Input: part model. Units: mm. Frame: model coordinates. A direction names the side the tool comes from. Coordinates: 2 decimals unless noted, no trailing zeros. Loops run counter-clockwise (first coordinate to the right, second up) from the corner with the lowest first, then second, coordinate; pieces in that order, holes last.
Item 1: Section A-A on z = 20.5. Return loops of the section in (x, y), and give its area (3 significant figures).
Item 2: Reachability of faces 4 (the cylindrical face through (9.573, -0.761, -150.211)), 5 (the flat face through (5, -16, 22)), 6 (the flat face through (5, -16, -112)), 7 (the flat face through (5, -16, -172)), 8 (the flat face through (14, -4, -21)) from +Z, -Z, +X, -X, +Y, -Y: full face, straight path, thin tool, end or side. Return the list, or none.
Item 3: Contact query for flat-ended pins moving along their axis: P1, Ø5, axis at y = -11.5, z = -102.5, coming from the +X side; P2, Ø3.5, axis at y = -18.5, z = -37.5, coming from the -X side; P3, Ø12.5, axis at x = 13, z = -49, coming from the -Y side; P4, Ø2.5, axis at y = -18, z = -54.5, coming from the +X side. Output: stop coordinate, or through.
Item 4: Ray query, line 1 along Y through (x, z) = (2.8, -95.5); line 2 along Y through (x, z) = (10, -54.5); line 3 along Y through (x, z) = (10.75, -92). Return the intervals inside material, ascending.
Item 5: Pull-direction query (Z, two-part tool) for faces 1 (the flat face through (19.289, -5.437, -73.509)), 2 (the cylindrical face through (7.1, -3.25, -56.3)), 3 (the flat face through (14, -4, 21)); classes: released by +Z, released by -Z, zero draft, split by the parting line, or undercut.
Item 6: Section C-C on z = -103. Return loops of the section in (x, y).
Item 7: Section D-D on x = 18.75. Return loops of the section in (y, z), and give its area (3 significant figures).
Item 8: Section B-B on y = -12.75. Return loops of the section in (x, z) (3 decimals).
```python
from build123d import *
from OCP.BRepFilletAPI import BRepFilletAPI_MakeChamfer

# Parameters (mm, degrees)
BOSS_EXTRUDE1_DEPTH     = 10
BOSS_EXTRUDE2_DEPTH     = 12
CUT_EXTRUDE3_DEPTH      = 6
CUT_EXTRUDE3_DEPTH_BACK = 14
SKETCH7_R               = 1.95
SKETCH8_R               = 1.95
CUT_EXTRUDE4_DEPTH      = 4
SKETCH9_R               = 1.5
CUT_EXTRUDE5_DEPTH      = 4
LPATTERN1_COUNT         = 2
LPATTERN1_PITCH         = 75
CHAMFER2_SIZE           = 5.5
CHAMFER2_SIZE2          = 9
CHAMFER3_SIZE           = 7
CHAMFER3_SIZE2          = 2
LPATTERN2_COUNT         = 3
LPATTERN2_PITCH         = 75


with BuildPart() as part:
    # Sketch1 → Boss-Extrude1 (new body)
    with BuildSketch(Plane(origin=(0, 0, 0), x_dir=(1, 0, 0), z_dir=(0, 1, 0))):
        with BuildLine():
            Line((0, -8.075), (0, -31.5))
            Line((0, -31.5), (22, -31.5))
            Line((22, -31.5), (22, 181.5))
            Line((22, 181.5), (0, 181.5))
            Line((0, 181.5), (0, 158.075))
            ThreePointArc((0, 158.075), (8.075, 150), (0, 141.925))
            Line((0, 141.925), (0, 83.075))
            ThreePointArc((0, 83.075), (8.075, 75), (0, 66.925))
            Line((0, 66.925), (0, 8.075))
            ThreePointArc((0, 8.075), (8.075, 0), (0, -8.075))
        make_face()
    extrude(amount=-BOSS_EXTRUDE1_DEPTH)

    # Sketch3 → Boss-Extrude2 (add)
    with BuildSketch(Plane.XZ.offset(10)):
        with BuildLine():
            Line((0, -181.5), (0, -158.075))
            ThreePointArc((0, -158.075), (8.075, -150), (0, -141.925))
            Line((0, -141.925), (0, -83.075))
            ThreePointArc((0, -83.075), (8.075, -75), (0, -66.925))
            Line((0, -66.925), (0, -8.075))
            ThreePointArc((0, -8.075), (8.075, 0), (0, 8.075))
            Line((0, 8.075), (0, 31.5))
            Line((0, 31.5), (5, 31.5))
            Line((5, 31.5), (5, 12.081209583))
            ThreePointArc((5, 12.081209583), (13.075, 0), (5, -12.081209583))
            Line((5, -12.081209583), (5, -62.918790417))
            ThreePointArc((5, -62.918790417), (13.075, -75), (5, -87.081209583))
            Line((5, -87.081209583), (5, -137.918790417))
            ThreePointArc((5, -137.918790417), (13.075, -150), (5, -162.081209583))
            Line((5, -162.081209583), (5, -181.5))
            Line((5, -181.5), (0, -181.5))
        make_face()
    extrude(amount=BOSS_EXTRUDE2_DEPTH)

    # Sketch7 → Cut-Extrude3 (cut, two sides: drawn at the far end of the back side and taken through both)
    with BuildSketch(Plane.ZY.offset(-CUT_EXTRUDE3_DEPTH_BACK)):
        with Locations((-170.5, -4)):
            Circle(SKETCH7_R)
        with Locations((-170.5, -18)):
            Circle(SKETCH7_R)
        with Locations(Location((-129.5, -4, 0), (0, 0, 180))):
            Circle(SKETCH7_R)
        with Locations((-129.5, -18)):
            Circle(SKETCH7_R)
        with Locations((-95.5, -4)):
            Circle(SKETCH7_R)
        with Locations(Location((-54.5, -4, 0), (0, 0, 180))):
            Circle(SKETCH7_R)
        with Locations((-54.5, -18)):
            Circle(SKETCH7_R)
        with Locations((-95.5, -18)):
            Circle(SKETCH7_R)
        with Locations((-20.5, -4)):
            Circle(SKETCH7_R)
        with Locations(Location((20.5, -4, 0), (0, 0, 180))):
            Circle(SKETCH7_R)
        with Locations((20.5, -18)):
            Circle(SKETCH7_R)
        with Locations((-20.5, -18)):
            Circle(SKETCH7_R)
    extrude(amount=CUT_EXTRUDE3_DEPTH + CUT_EXTRUDE3_DEPTH_BACK, mode=Mode.SUBTRACT)

    # Sketch8 → Cut-Extrude4 (cut)
    with BuildSketch(Plane.ZY):
        with Locations((-112.5, -18.5)):
            Circle(SKETCH8_R)
    cut_extrude4 = extrude(amount=-CUT_EXTRUDE4_DEPTH, mode=Mode.SUBTRACT)

    # Sketch9 → Cut-Extrude5 (cut)
    with BuildSketch(Plane.ZY.offset(-4)):
        with Locations((-112.5, -18.5)):
            Circle(SKETCH9_R)
    cut_extrude5 = extrude(amount=-CUT_EXTRUDE5_DEPTH, mode=Mode.SUBTRACT)

    # LPattern1: Cut-Extrude4, Cut-Extrude5 ×2
    with Locations(*[(0, 0, i * LPATTERN1_PITCH) for i in range(1, LPATTERN1_COUNT)]):
        add(cut_extrude4, mode=Mode.SUBTRACT)
        add(cut_extrude5, mode=Mode.SUBTRACT)

    # Chamfer2
    chamfer2_edges = [part.edges().sort_by_distance(p)[0] for p in [
        (22, -10, -75),
    ]]
    chamfer2_side = [part.faces().sort_by_distance(p)[0] for p in [
        (14.183508734, -10, -75),
    ]]
    chamfer(chamfer2_edges, length=CHAMFER2_SIZE, length2=CHAMFER2_SIZE2, reference=chamfer2_side[0])

    # Chamfer3: one chamfer whose edges measure the first distance from different faces: ONE call of the kernel's chamfer builder (chamfer() names one face for all edges)
    chamfer3_edges_1 = [part.edges().sort_by_distance(p)[0] for p in [
        (8.075, -22, 0),
    ]]
    chamfer3_side_1 = [part.faces().sort_by_distance(p)[0] for p in [
        (8.075, -11, 0),
    ]]
    chamfer3_edges_2 = [part.edges().sort_by_distance(p)[0] for p in [
        (8.075, -22, -75),
    ]]
    chamfer3_side_2 = [part.faces().sort_by_distance(p)[0] for p in [
        (8.075, -11, -75),
    ]]
    chamfer3_edges_3 = [part.edges().sort_by_distance(p)[0] for p in [
        (8.075, -22, -150),
    ]]
    chamfer3_side_3 = [part.faces().sort_by_distance(p)[0] for p in [
        (8.075, -11, -150),
    ]]
    chamfer3 = BRepFilletAPI_MakeChamfer(part.part.solid().wrapped)
    for e in chamfer3_edges_1:
        chamfer3.Add(CHAMFER3_SIZE, CHAMFER3_SIZE2, e.wrapped, chamfer3_side_1[0].wrapped)  # the first distance lies on this face
    for e in chamfer3_edges_2:
        chamfer3.Add(CHAMFER3_SIZE, CHAMFER3_SIZE2, e.wrapped, chamfer3_side_2[0].wrapped)  # the first distance lies on this face
    for e in chamfer3_edges_3:
        chamfer3.Add(CHAMFER3_SIZE, CHAMFER3_SIZE2, e.wrapped, chamfer3_side_3[0].wrapped)  # the first distance lies on this face
    add(Compound.cast(chamfer3.Shape()), mode=Mode.REPLACE)

    # Sketch10 → Cut-Revolve1 (revolve, cut)
    with BuildSketch(Plane.ZY):
        with BuildLine():
            Line((-159.575, 1.581763394), (-159.575, -1.5))
            ThreePointArc((-159.575, -1.5), (-157.014339828, -2.560660172), (-158.075, 0))
            Line((-158.075, 0), (-159.575, 1.581763394))
        make_face()
    cut_revolve1 = revolve(axis=Axis((0, 2.197765982, -150), (0, -1, 0)), mode=Mode.SUBTRACT)

    # LPattern2: Cut-Revolve1 ×3
    with Locations(*[(0, 0, i * LPATTERN2_PITCH) for i in range(1, LPATTERN2_COUNT)]):
        add(cut_revolve1, mode=Mode.SUBTRACT)


solid = part.part
```
Results found:
1. outline: (0, -22) - (5, -22) - (5, -19.95) - (0, -19.95) - close; (0, -16.05) - (5, -16.05) - (5, -10) - (16.5, -10) - (22, -1) - (22, 0) - (0, 0) - (0, -2.05) - (14, -2.05) - (14, -5.95) - (0, -5.95) - close
1. area: 181 mm2
2. face 4: -X, +Y
2. face 5: +Z, +X, -Y
2. face 6: +X, -Y
2. face 7: -Z, +X, -Y
2. face 8: -X
3. P1: stops at x = 17.11
3. P2: stops at x = 4
3. P3: stops at y = -10
3. P4: passes through
4. line 1: y = -22 to -19.95, -16.05 to -5.95, -2.05 to 0
4. line 2: y = -10 to -5.95, -2.05 to 0
4. line 3: y = -10 to 0
5. face 1: zero draft
5. face 2: undercut
5. face 3: undercut
6. outline: (0, -22) - (5, -22) - (5, -10) - (16.5, -10) - (22, -1) - (22, 0) - (0, 0) - close
7. outline: (-6.32, -181.5) - (0, -181.5) - (0, 31.5) - (-6.32, 31.5) - close
7. area: 1,350 mm2
8. outline: (0, -181.5) - (5, -181.5) - (5, -162.081) arc R13.075 ccw to (5, -137.919) - (5, -87.081) arc R13.075 ccw to (5, -62.919) - (5, -12.081) arc R13.075 ccw to (5, 12.081) - (5, 31.5) - (0, 31.5) - (0, 8.075) arc R8.075 cw to (0, -8.075) - (0, -66.925) arc R8.075 cw to (0, -83.075) - (0, -141.925) arc R8.075 cw to (0, -158.075) - close
